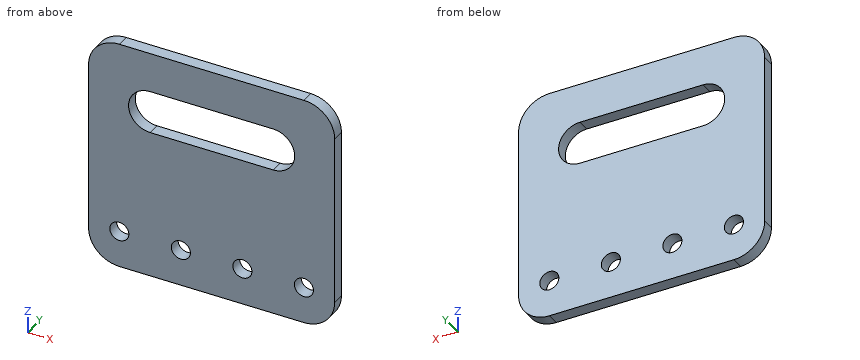
from build123d import *

# Parameters (mm, degrees)
F0_W     = 200
F0_H     = 190
F1_DEPTH = 10
F3_D     = 15.5
F4_R     = 25


with BuildPart() as f1:
    # F0 (on Front) → F1 (new body)
    with BuildSketch(Plane.XZ):
        Rectangle(F0_W, F0_H)
        with BuildLine():
            ThreePointArc((-50, 27.5), (-67.5, 45), (-50, 62.5))
            Line((-50, 62.5), (50, 62.5))
            ThreePointArc((50, 62.5), (67.5, 45), (50, 27.5))
            Line((50, 27.5), (-50, 27.5))
        make_face(mode=Mode.SUBTRACT)
    extrude(amount=F1_DEPTH)

    # F3 (through all)
    with Locations(Plane.XZ.offset(10)):
        with Locations((-75, -65), (-25, -65), (25, -65), (75, -65)):
            Hole(F3_D / 2)

    # F4
    f4_edges = [f1.edges().sort_by_distance(p)[0] for p in [
        (100, -5, 95),
        (-100, -5, 95),
        (100, -5, -95),
        (-100, -5, -95),
    ]]
    fillet(f4_edges, radius=F4_R)


solid = f1.part
CAD build for the part. Positions are in the model's coordinates, mm. Coordinates: 2 decimals unless noted, no trailing zeros. Write each loop counter-clockwise with the first axis right and the second up, starting at its lowest first coordinate (ties: lowest second). Pieces come first, ordered by that corner, then holes. Notation, with made-up numbers: (18, -1.5) - (26, -1.5) arc R20 cw to (26, 20.5) - close; hole circle Ø3 at (29, -23.5). An arc over 180 degrees is marked (long way). Use a Markdown table: item, result. Add a question column.
Item 1: Band-saw the part on B-B, the plane x = -25. Give the cut face in (y, z), and give its area (4 significant figures).
Item 2: Band-saw the part on D-D, the plane z = -65. Give the cut face in (x, y), and give its area (3 significant figures).
Item 3: Band-saw the part on A-A, the plane z = 45. Give the cut face in (x, y), and give its area (3 significant figures).
Item 4: Drill centre lines: L1, parallel to Z at x = 25, y = -3.25; L2, parallel to Z at x = 75, y = -5; L3, parallel to Z at x = -6.5, y = -9. Where is each one in solid material? Low to high. Write a range as from..to.
Item 5: Flat gauge pin, fed straight in: pin 1 (6 mm diameter, centred on y = -7, z = -70.5, fed in from -X). Where does the tip first touch, or does it go through?
Item 6: Band-saw the part on C-C, the plane y = -1.5. Give the cut face in (x, z), and give its area (3 significant figures).
Numbers:
| question | item | result |
|---|---|---|
| 1 | outline | (-10, -95) - (0, -95) - (0, -72.75) - (-10, -72.75) - close; (-10, -57.25) - (0, -57.25) - (0, 27.5) - (-10, 27.5) - close; (-10, 62.5) - (0, 62.5) - (0, 95) - (-10, 95) - close |
| 1 | area | 1,395 mm2 |
| 2 | outline | (-100, -10) - (-82.75, -10) - (-82.75, 0) - (-100, 0) - close; (-67.25, -10) - (-32.75, -10) - (-32.75, 0) - (-67.25, 0) - close; (-17.25, -10) - (17.25, -10) - (17.25, 0) - (-17.25, 0) - close; (32.75, -10) - (67.25, -10) - (67.25, 0) - (32.75, 0) - close; (82.75, -10) - (100, -10) - (100, 0) - (82.75, 0) - close |
| 2 | area | 1,380 mm2 |
| 3 | outline | (-100, -10) - (-67.5, -10) - (-67.5, 0) - (-100, 0) - close; (67.5, -10) - (100, -10) - (100, 0) - (67.5, 0) - close |
| 3 | area | 650 mm2 |
| 4 | L1 | -95..-72.75, -57.25..27.5, 62.5..95 |
| 4 | L2 | -95..-72.75, -57.25..95 |
| 4 | L3 | -95..27.5, 62.5..95 |
| 5 | pin 1 | x = -100 |
| 6 | outline | (-100, -70) arc R25 ccw to (-75, -95) - (75, -95) arc R25 ccw to (100, -70) - (100, 70) arc R25 ccw to (75, 95) - (-75, 95) arc R25 ccw to (-100, 70) - close; hole circle Ø15.5 at (-75, -65); hole (-50, 27.5) - (50, 27.5) arc R17.5 ccw to (50, 62.5) - (-50, 62.5) arc R17.5 ccw to start; hole circle Ø15.5 at (-25, -65); hole circle Ø15.5 at (25, -65); hole circle Ø15.5 at (75, -65) |
| 6 | area | 32,200 mm2 |
